Autodesk Inventor part; units mm, degrees
ref_plane "WorkPlane1" through (0, 0, 0) normal (0, 0, 1) x (1, 0, 0)
ref_plane "Work Plane2" through (0, 0, -2) normal (0, 0, 1) x (1, 0, 0)
ref_plane "WorkPlane2" through (0, 0, 1) normal (0, 0, 1) x (1, 0, 0)
ref_plane "WorkPlane1" through (0, 0, 0) normal (0, 0, 1) x (1, 0, 0)
ref_plane "Work Plane2" through (0, 0, -2) normal (0, 0, 1) x (1, 0, 0)
ref_plane "WorkPlane2" through (0, 0, 1) normal (0, 0, 1) x (1, 0, 0)
sketch "Sketch1" plane through (0, 0, 0) normal (0, 0, 1) x (1, 0, 0)
  point P0 (0, 0)
sketch "Sketch2" plane through (0, 0, 0) normal (0, 0, 1) x (1, 0, 0)
  line L0 (6.5, -27.1007) -> (5.6878, -23.5434)
  arc A0 (9.3615, -21.348) -> (5.6878, -23.5434) centre (7.8813, -23.0425) ccw
  line L1 (9.3615, -21.348) -> (11.8371, -23.5105)
  arc A1 (11.8371, -23.5105) -> (-11.8371, -23.5105) centre (0, 0) ccw
  line L2 (-9.3615, -21.348) -> (-11.8371, -23.5105)
  arc A2 (-5.6878, -23.5434) -> (-9.3615, -21.348) centre (-7.8813, -23.0425) ccw
  line L3 (-6.5, -27.1007) -> (-5.6878, -23.5434)
  arc A3 (6.5, -27.1007) -> (-6.5, -27.1007) centre (0, 1.3667) ccw
  line L4 (0, 1.3667) -> (-6.5, -27.1007) construction
  line L5 (0, 1.3667) -> (6.5, -27.1007) construction
  dimension "d2" = 29.2
  dimension "d4" = 0
  dimension "d6" = 26.3222
  dimension "d8" = 1.3667
  dimension "d10" = 6.5
  dimension "d12" = 6.5
  dimension "d14" = 2.25
  dimension "d16" = 2.25
  dimension "d18" = 25.65
  dimension "d20" = 25.65
  dimension "d22" = 36
  dimension "d24" = 36
extrude "Extrusion1" add sketch "Sketch2" along normal blind 2
sketch "Sketch3" plane through (0, 0, 2) normal (0, 0, 1) x (1, 0, 0)
  arc A0 (-5.6878, -23.5434) -> (-9.3615, -21.348) centre (-7.8813, -23.0425) ccw
hole "Hole1" at (-7.8813, -23.0425, 2) direction (0, 0, -1) diameter 2.5 end through all
sketch "Sketch4" plane through (0, 0, 2) normal (0, 0, 1) x (1, 0, 0)
  arc A0 (9.3615, -21.348) -> (5.6878, -23.5434) centre (7.8813, -23.0425) ccw
hole "Hole2" at (7.8813, -23.0425, 2) direction (0, 0, -1) diameter 2.5 end through all
equation "\"d29\" = Diam5"
equation "\"d36\" = Diam5"
equation "\"d2\" = 0.5 * Diam2"
equation "\"d6\" = 0.5 * msp_dd1"
equation "\"d8\" = -0.5 * msp_dd1 + 0.5 * Diam2 - 0.222222 * ParA"
equation "\"d10\" = 2.6 * Diam5"
equation "\"d12\" = 2.6 * Diam5"
equation "\"d14\" = 0.9 * Diam5"
equation "\"d16\" = 0.9 * Diam5"
equation "\"d18\" = 1.3 * Diam5 + 0.5 * Diam2 - ParA"
equation "\"d20\" = 1.3 * Diam5 + 0.5 * Diam2 - ParA"
equation "\"d25\" = ParS"
equation "\"Diam5\" = 2.5"
equation "\"ParA\" = 6.8"
equation "\"ParS\" = 2"
equation "\"Diam2\" = 58.4"
equation "\"msp_dd1\" = -b + Diam2 - 0.111111 * ParA"
equation "\"msp_pom\" = 0.5 * Diam2 - b"
equation "\"TEMPLATE\" = 1.2345"
properties part number "ANSI B 27.7M - 3BMI-55" material "Steel, Mild"
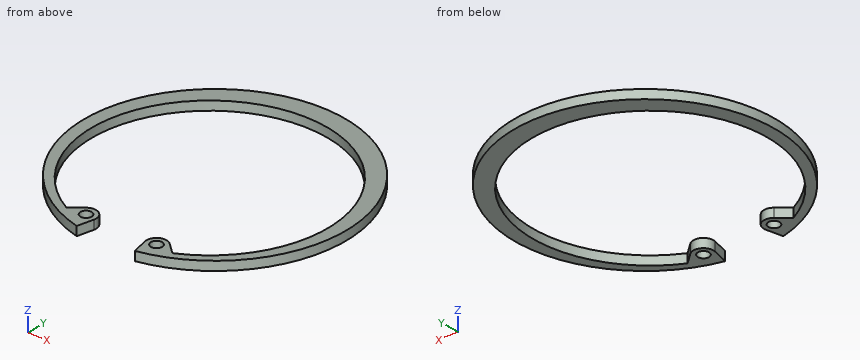
Geometry check sheet. Reference: the model listing, model coordinates, mm. Coordinates: 2 decimals unless noted, no trailing zeros. Order: outer loops, then holes, each group sorted by start corner. A loop starts at its lowest first (then second) coordinate and runs counter-clockwise, first axis right, second up.
Item 1: Section check B-B (x = 20.5). Enter the section's corners in (y, z).
Item 2: Section check C-C (z = 1). Enter the section's corners in (x, y).
Item 3: Section check A-A (y = -8.5). Enter the section's corners in (x, z), plus the area to 3 significant figures.
Item 4: Scan lines: line 1 along X through (y, z) = (-24, 0.3); line 2 along Y through (x, z) = (0, 0.6); line 3 along Y through (x, z) = (-23.5, 1.7). Record each from-to range of solid material in increasing order.
Item 5: Section check D-D (x = 0). Enter the section's corners in (y, z), plus the area to 3 significant figures.
Item 6: Depth check by flat-ended pin: pin 1 (6 mm diameter, centred on x = 9, y = 19.5, fed in from -Z). Enter the tip coordinate at first touch or a pass-through.
Check sheet entries:
1. outline: (-19.43, 0) - (-16.51, 0) - (-16.51, 2) - (-19.43, 2) - close; (16.51, 0) - (22.16, 0) - (22.16, 2) - (16.51, 2) - close
2. outline: (-11.84, -23.51) arc R26.32 cw (long way) to (11.84, -23.51) - (9.36, -21.35) arc R2.25 ccw to (5.69, -23.54) - (6.5, -27.1) arc R29.2 ccw (long way) to (-6.5, -27.1) - (-5.69, -23.54) arc R2.25 ccw to (-9.36, -21.35) - close; hole circle Ø2.5 at (-7.88, -23.04); hole circle Ø2.5 at (7.88, -23.04)
3. outline: (-27.48, 0) - (-24.91, 0) - (-24.91, 2) - (-27.48, 2) - close; (24.91, 0) - (27.48, 0) - (27.48, 2) - (24.91, 2) - close
3. area: 10.3 mm2
4. line 1: x = -14.46 to -8.68, -7.08 to -5.79, 5.79 to 7.08, 8.68 to 14.46
4. line 2: y = 26.32 to 30.57
4. line 3: y = -15.97 to -11.86, 11.86 to 18.7
5. outline: (26.32, 0) - (30.57, 0) - (30.57, 2) - (26.32, 2) - close
5. area: 8.49 mm2
6. pin 1: passes through
